Geometry check sheet. Reference: the model listing, model coordinates, mm. Round coordinates to 2 decimals unless told otherwise and drop trailing zeros. Loops run counter-clockwise (first coordinate to the right, second up) from the corner with the lowest first, then second, coordinate; pieces in that order, holes last. Notation, with made-up numbers: (64.25, -40) - (88.25, -40) arc R25 ccw to (88.25, -21) - close; hole circle Ø9 at (35, 4.5). An arc over 180 degrees is marked (long way). Write item = value, one per line.
```python
from build123d import *

# Parameters (mm, degrees)
SKETCH1_W           = 25
SKETCH1_H           = 25
BOSS_EXTRUDE1_DEPTH = 12
SKETCH2_R           = 1.5
BOSS_EXTRUDE2_DEPTH = 15
SKETCH3_R           = 1.5


with BuildPart() as part:
    # Sketch1 → Boss-Extrude1 (new body)
    with BuildSketch(Plane(origin=(0, 0, 0), x_dir=(1, 0, 0), z_dir=(0, 1, 0))):
        Rectangle(SKETCH1_W, SKETCH1_H)
    extrude(amount=BOSS_EXTRUDE1_DEPTH)

    # Sketch2 → Boss-Extrude2 (add)
    with BuildSketch(Plane(origin=(0, 12, 0), x_dir=(1, 0, 0), z_dir=(0, 1, 0))):
        Circle(SKETCH2_R)
    extrude(amount=BOSS_EXTRUDE2_DEPTH)

    # Sketch3 → Revolve1 (revolve)
    with BuildSketch(Plane(origin=(0, 31.999999906, 0), x_dir=(1, 0, 0), z_dir=(0, 1, 0))):
        with Locations((-5, 0)):
            Circle(SKETCH3_R)
    revolve(axis=Axis((0, 31.999999906, -13.75), (0, 0, 1)))


solid = part.part
```
(1) Mould release check, pull along Y, two halves, no side actions. Record for faces 1 (the cylindrical face through (1.43, 19.39, -0.45)), 2 (the flat face through (0, 0, 0)), 3 (the flat face through (-12.5, 6, 0)): pulls with the +Y half, pulls with the -Y half, needs draft (parallel to the pull), parting line crosses it, or undercut.
Answers follow:
face_1 = undercut
face_2 = pulls with the -Y half
face_3 = needs draft
(2) Section check C-C (y = 20). Enter the section's corners in (x, z).
Answers follow:
outline = circle Ø3 at (0, 0)
(3) Section check B-B (x = 0). Enter the section's corners in (y, z).
Answers follow:
outline = (0, -12.5) - (12, -12.5) - (12, -1.5) - (27, -1.5) arc R1.5 ccw to (27, 1.5) - (12, 1.5) - (12, 12.5) - (0, 12.5) - close; circle Ø3 at (37, 0)
(4) Gauge pin test, flat ends, axial feed: pin 1 (10 mm diameter, centred on x = 2.5, y = 18.5, fed in from +Z); pin 2 (12 mm diameter, centred on x = -7.5, z = -8.5, fed in from +Y); pin 3 (1.5 mm diameter, centred on x = 3, y = 15.5, fed in from -Z); pin 4 (1 mm diameter, centred on y = 21.5, z = -0.5, fed in from +X). Record the tip position at first contact, or that the pin passes through.
Answers follow:
pin_1 = 1.5
pin_2 = 12
pin_3 = through
pin_4 = 1.5
(5) Section check D-D (x = -10.25). Enter the section's corners in (y, z).
Answers follow:
outline = (0, -12.5) - (12, -12.5) - (12, 12.5) - (0, 12.5) - close
(6) Section check A-A (z = 0). Enter the section's corners in (x, y).
Answers follow:
outline = (-12.5, 0) - (12.5, 0) - (12.5, 12) - (1.5, 12) - (1.5, 25.68) arc R6.5 ccw (long way) to (-1.5, 25.68) - (-1.5, 12) - (-12.5, 12) - close; hole circle Ø7 at (0, 32)
(7) Scan lines: L1, parallel to Y at x = -1.75, z = 2.25; L2, parallel to Z at x = -1, y = 37; L3, parallel to Y at x = 4.25, z = 0. Record each from-to range of solid material in increasing order. Write a range as [from, to].
Answers follow:
L1 = [0, 12]
L2 = [-1.5, 1.5]
L3 = [0, 12], [27.08, 36.92]
